from build123d import *

# Parameters (mm, degrees)
BOSS_EXTRUDE1_DEPTH      = 40.5
BOSS_EXTRUDE1_DEPTH_BACK = 40.5
SKETCH1_R                = 7
CUT_EXTRUDE1_START       = -67.5
SKETCH2_R                = 12.499999991
SKETCH2_R_2              = 7
SKETCH2_R_3              = 12.5
CUT_EXTRUDE1_DEPTH       = 54
BOSS_EXTRUDE2_DEPTH      = 49.000000379
CUT_EXTRUDE2_START       = -14.999999621
SKETCH4_R                = 7.499999993
SKETCH4_R_2              = 1.499999993
CUT_EXTRUDE2_DEPTH       = 14.999999621
SKETCH5_R                = 6.999999993
CUT_EXTRUDE3_DEPTH       = 221.420620892
BOSS_EXTRUDE3_DEPTH      = 7
CUT_EXTRUDE6_START       = 10
SKETCH7_R                = 14.249999993
SKETCH7_R_2              = 6.999999993
CUT_EXTRUDE6_DEPTH       = 211.420621005


# Read off the part's stored shape, not the designer's step: Boss-Extrude3
with BuildPart() as part:
    # Sketch1 → Boss-Extrude1 (new, two sides: drawn at the far end of the back side and taken through both)
    with BuildSketch(Plane.XY.offset(-BOSS_EXTRUDE1_DEPTH_BACK)):
        with BuildLine():
            ThreePointArc((101.284221271, -32.899999986), (83.546912911, -43.395194612), (65.376921076, -33.668293007))
            ThreePointArc((65.376921076, -33.668293007), (33.566126775, -31.096638376), (39.782202113, -62.4))
            Line((39.782202113, -62.4), (207.000000276, -62.4))
            Line((207.000000276, -62.4), (207.000000276, -47.400000379))
            Line((207.000000276, -47.400000379), (160, -47.400000379))
            Line((160, -47.400000379), (160, 1.6))
            Line((160, 1.6), (152, 1.6))
            Line((152, 1.6), (145.25, -13.4))
            Line((145.25, -13.4), (112.542551513, -13.4))
            Line((112.542551513, -13.4), (101.284221271, -32.899999986))
        make_face()
        with Locations((142, -31.4)):
            Circle(SKETCH1_R, mode=Mode.SUBTRACT)
        with Locations((48.5, -44.4)):
            Circle(SKETCH1_R, mode=Mode.SUBTRACT)
    extrude(amount=BOSS_EXTRUDE1_DEPTH + BOSS_EXTRUDE1_DEPTH_BACK)

    # Sketch2 → Cut-Extrude1 (cut)
    # profile 1 of 4: a face of its own
    with BuildSketch(Plane.XY.offset(40.5).offset(CUT_EXTRUDE1_START)):
        with Locations((142, -31.4)):
            Circle(SKETCH2_R)
        with Locations(Location((142, -31.4, 0), (0, 0, 180))):
            Circle(SKETCH2_R_2, mode=Mode.SUBTRACT)
    # profile 2 of 4: a face of its own
    with BuildSketch(Plane.XY.offset(40.5).offset(CUT_EXTRUDE1_START)):
        with BuildLine():
            Line((61, -44.4), (61, -28.787505004))
            ThreePointArc((61, -28.787505004), (39.839745962, -26.372243623), (28.5, -44.4))
            ThreePointArc((28.5, -44.4), (29.628726859, -51.023824427), (32.887505004, -56.9))
            Line((32.887505004, -56.9), (48.5, -56.9))
            ThreePointArc((48.5, -56.9), (39.661165235, -35.561165235), (61, -44.4))
        make_face()
    # profile 3 of 4: a face of its own
    with BuildSketch(Plane.XY.offset(40.5).offset(CUT_EXTRUDE1_START)):
        with Locations((48.5, -44.4)):
            Circle(SKETCH2_R_3)
        with Locations(Location((48.5, -44.4, 0), (0, 0, 180))):
            Circle(SKETCH2_R_2, mode=Mode.SUBTRACT)
    # profile 4 of 4: a face of its own
    with BuildSketch(Plane.XY.offset(40.5).offset(CUT_EXTRUDE1_START)):
        with BuildLine():
            ThreePointArc((101.284221271, -32.899999986), (100.261640945, -34.499533541), (99.0987841, -36.000180759))
            Line((99.0987841, -36.000180759), (139.674860989, -43.681845488))
            ThreePointArc((139.674860991, -43.681845479), (134.025485527, -21.774143224), (154.499999991, -31.4))
            Line((154.5, -31.4), (154.5, -13.4))
            Line((154.5, -13.4), (145.25, -13.4))
            Line((145.25, -13.4), (112.542551513, -13.4))
            Line((112.542551513, -13.4), (101.284221271, -32.899999986))
        make_face()
    extrude(amount=CUT_EXTRUDE1_DEPTH, mode=Mode.SUBTRACT)

    # Sketch3 → Boss-Extrude2 (add)
    with BuildSketch(Plane(origin=(0, -47.400000379, 0), x_dir=(1, 0, 0), z_dir=(0, 1, 0))):
        with BuildLine():
            Line((198.298990268, 40.5), (160, 40.5))
            Line((160, 40.5), (160, 24.330126958))
            ThreePointArc((160, 24.330126958), (197.5, 20), (160, 15.669873042))
            Line((160, 15.669873042), (160, -15.669873042))
            ThreePointArc((160, -15.669873042), (197.5, -20), (160, -24.330126958))
            Line((160, -24.330126958), (160, -40.5))
            Line((160, -40.5), (198.298990268, -40.5))
            ThreePointArc((198.298990268, -40.5), (204.734721686, -31.135052483), (207.000000277, -20))
            Line((207.000000276, -20), (207.000000276, 20))
            ThreePointArc((207.000000277, 20), (204.734721686, 31.135052483), (198.298990268, 40.5))
        make_face()
    extrude(amount=BOSS_EXTRUDE2_DEPTH)

    # Sketch4 → Cut-Extrude2 (cut)
    with BuildSketch(Plane(origin=(0, -47.400000379, 0), x_dir=(1, 0, 0), z_dir=(0, 1, 0)).offset(CUT_EXTRUDE2_START)):
        with BuildLine():
            Line((207.000000276, 20), (207.000000276, 40.5))
            Line((207.000000276, 40.5), (198.298990268, 40.5))
            ThreePointArc((198.298990268, 40.5), (204.734721686, 31.135052483), (207.000000277, 20))
        make_face()
        with BuildLine():
            Line((207.000000276, -40.5), (207.000000276, -20))
            ThreePointArc((207.000000277, -20), (204.734721686, -31.135052483), (198.298990268, -40.5))
            Line((198.298990268, -40.5), (207.000000276, -40.5))
        make_face()
        with Locations(Location((171.500000007, -20, 0), (0, 0, 180))):
            Circle(SKETCH4_R)
        with Locations(Location((171.500000007, 20, 0), (0, 0, 180))):
            Circle(SKETCH4_R)
        with Locations(Location((178.500000007, 4.5, 0), (0, 0, 180))):
            Circle(SKETCH4_R_2)
        with Locations(Location((165.076606249, 12.25, 0), (0, 0, 180))):
            Circle(SKETCH4_R_2)
        with Locations(Location((191.923393766, 12.25, 0), (0, 0, 180))):
            Circle(SKETCH4_R_2)
        with Locations(Location((191.923393766, 27.75, 0), (0, 0, 180))):
            Circle(SKETCH4_R_2)
        with Locations(Location((178.500000007, 35.5, 0), (0, 0, 180))):
            Circle(SKETCH4_R_2)
        with Locations(Location((165.076606249, 27.75, 0), (0, 0, 180))):
            Circle(SKETCH4_R_2)
        with Locations(Location((165.076606249, -12.25, 0), (0, 0, 180))):
            Circle(SKETCH4_R_2)
        with Locations(Location((178.500000007, -4.5, 0), (0, 0, 180))):
            Circle(SKETCH4_R_2)
        with Locations(Location((191.923393766, -12.25, 0), (0, 0, 180))):
            Circle(SKETCH4_R_2)
        with Locations(Location((191.923393766, -27.75, 0), (0, 0, 180))):
            Circle(SKETCH4_R_2)
        with Locations(Location((178.500000007, -35.5, 0), (0, 0, 180))):
            Circle(SKETCH4_R_2)
        with Locations(Location((165.076606249, -27.75, 0), (0, 0, 180))):
            Circle(SKETCH4_R_2)
    extrude(amount=CUT_EXTRUDE2_DEPTH, mode=Mode.SUBTRACT)

    # Sketch5 → Cut-Extrude3 (cut, through all)
    with BuildSketch(Plane.XZ.offset(62.4)):
        with Locations((139.189011165, 0)):
            Circle(SKETCH5_R)
    extrude(amount=-CUT_EXTRUDE3_DEPTH, mode=Mode.SUBTRACT)

    # Boss-Extrude3 outline → Boss-Extrude3 (add)
    with BuildSketch(Plane.XZ.offset(62.4)):
        with BuildLine():
            ThreePointArc((139.189011157, 40), (99.189011157, 0), (139.189011157, -40))
            add(Edge.make_bspline(
                [(139.189011157, -40), (146.82843448, -40), (162.107281125, -38.078486158), (176.778501223, -31.90101694), (183.851500427, -26.99841863), (185.64679387, -25.589452029), (186.4885893, -24.893504667), (187.107516855, -24.363583077), (187.51172734, -24.005038173), (187.711696887, -23.824463012)],
                knots=[1.570796327, 1.570796327, 1.570796327, 1.570796327, 1.963495408, 2.35619449, 2.445236625, 2.478897191, 2.495727474, 2.512557757, 2.52938804, 2.52938804, 2.52938804, 2.52938804], degree=3))
            Line((187.711696887, -23.824463012), (187.711696887, 23.824463012))
            add(Edge.make_bspline(
                [(187.711696887, 23.824463012), (187.51172734, 24.005038173), (187.107516855, 24.363583077), (186.4885893, 24.893504667), (185.64679387, 25.589452029), (183.851500427, 26.99841863), (176.778501223, 31.90101694), (162.107281125, 38.078486158), (146.82843448, 40), (139.189011157, 40)],
                knots=[3.753797267, 3.753797267, 3.753797267, 3.753797267, 3.77062755, 3.787457833, 3.804288116, 3.837948682, 3.926990817, 4.319689899, 4.71238898, 4.71238898, 4.71238898, 4.71238898], degree=3))
        make_face()
        with BuildLine():
            add(Edge.make_bspline(
                [(139.189011157, -35), (166.137629731, -35), (182.711696887, -21.525865932)],
                knots=[1.570796327, 1.570796327, 1.570796327, 2.479175311, 2.479175311, 2.479175311], degree=2, weights=[1, 0.898616921, 1]))
            ThreePointArc((139.189011157, -35), (104.189011157, 0), (139.189011157, 35))
            add(Edge.make_bspline(
                [(182.711696887, 21.525865932), (166.137629731, 35), (139.189011157, 35)],
                knots=[3.804009997, 3.804009997, 3.804009997, 4.71238898, 4.71238898, 4.71238898], degree=2, weights=[1, 0.898616921, 1]))
            Line((182.711696887, 21.525865932), (182.711696887, -21.525865932))
        make_face(mode=Mode.SUBTRACT)
    extrude(amount=BOSS_EXTRUDE3_DEPTH)

    # Sketch7 → Cut-Extrude6 (cut, through all)
    # profile 1 of 2: a face of its own
    with BuildSketch(Plane(origin=(0, -62.4, 0), x_dir=(1, 0, 0), z_dir=(0, 1, 0)).offset(CUT_EXTRUDE6_START)):
        with Locations((139.189011165, 0)):
            Circle(SKETCH7_R)
        with Locations((139.189011165, 0)):
            Circle(SKETCH7_R_2, mode=Mode.SUBTRACT)
    # profile 2 of 2: a face of its own
    with BuildSketch(Plane(origin=(0, -62.4, 0), x_dir=(1, 0, 0), z_dir=(0, 1, 0)).offset(CUT_EXTRUDE6_START)):
        with Locations((139.189011165, 0)):
            Circle(SKETCH7_R_2)
    extrude(amount=CUT_EXTRUDE6_DEPTH, mode=Mode.SUBTRACT)


solid = part.part
Geometry: final body of the model. Coordinates: model frame, mm. A direction names the side the tool comes from. Round coordinates to 2 decimals unless told otherwise and drop trailing zeros. Order: outer loops, then holes, each group sorted by start corner. A loop starts at its lowest first (then second) coordinate and runs counter-clockwise, first axis right, second up.
Q1. Section C-C, the plane x = 110. Output: boundary loops of the cut face in (y, z).
Result sheet:
outline: (-69.4, -27.35) - (-62.4, -27.35) - (-62.4, -40.5) - (-17.8, -40.5) - (-17.8, -27) - (-38.06, -27) - (-38.06, 27) - (-17.8, 27) - (-17.8, 40.5) - (-62.4, 40.5) - (-62.4, 27.35) - (-69.4, 27.35) - (-69.4, 19.31) - (-62.4, 19.31) - (-62.4, -19.31) - (-69.4, -19.31) - close
Q2. Pin query (flat end, axial travel): pin 1 (4 mm diameter, centred on x = 191.92, z = 27.75, fed in from +Y); pin 2 (10 mm diameter, centred on x = 62.5, z = -2.5, fed in from +Y); pin 3 (4.5 mm diameter, centred on y = -29.5, z = -20.5, fed in from +X); pin 4 (4 mm diameter, centred on x = 191.92, z = -27.75, fed in from -Y). Return the tip coordinate at first contact, or that it passes through.
Result sheet:
pin 1: stops at y = -47.4
pin 2: stops at y = -28.79
pin 3: stops at x = 207
pin 4: stops at y = -62.4
Q3. Material intervals for probe 1 along Z at (x, y) = (171, -53); probe 2 along Z at (x, y) = (181.5, -17); probe 3 along X at (y, z) = (-34, -6), sorted ascending.
Result sheet:
probe 1: z = -40.5 to -27.48, -12.52 to 12.52, 27.48 to 40.5
probe 2: z = -40.5 to -38.76, -1.24 to 1.24, 38.76 to 40.5
probe 3: x = 61 to 65.59, 154.23 to 165.65, 191.35 to 207
Q4. Access query for faces 1 (the face through (129, -13.4, -34)), 2 (the face through (45, -37, 27)), 3 (the face through (183, -47.4, 20)), 4 (the face through (187.712, -66, 0)). Directions: +Z, -Z, +X, -X, +Y, -Y. A direction counts if a zero-diameter tool reaches every point of the face in a straight line with its end or side. Return the directions, or none.
Result sheet:
face 1: +Z, -Z, -X, +Y
face 2: -X, +Y
face 3: +Y
face 4: +Z, -Z, +X, -Y
Q5. Section B-B, the plane y = -9. Output: boundary loops of the cut face in (x, z).
Result sheet:
outline: (147.23, -40.5) - (198.3, -40.5) arc R28.5 ccw to (207, -20) - (207, 20) arc R28.5 ccw to (198.3, 40.5) - (147.23, 40.5) - (147.23, 11.76) arc R14.25 cw to (147.23, -11.76) - close; hole (160, -24.33) arc R19 ccw (long way) to (160, -15.67) - close; hole (160, 15.67) arc R19 ccw (long way) to (160, 24.33) - close
Q6. Mould query, pull axis Y, two halves, no side actions, for faces 5 (the face through (143.2, -69.4, -35.4)), 6 (the face through (183, -47.4, -20)), 7 (the face through (154.5, -23, 0)). Classes: released by +Y, released by -Y, zero draft, split by the parting line, or undercut.
Result sheet:
face 5: released by -Y
face 6: released by +Y
face 7: undercut
Q7. Section A-A, the plane y = -59. Give the number of separate pieces and of enclosed holes in the cut face, and give its area (3 significant figures).
Result sheet:
separate pieces: 1
enclosed holes: 15
area: 13,200 mm2
